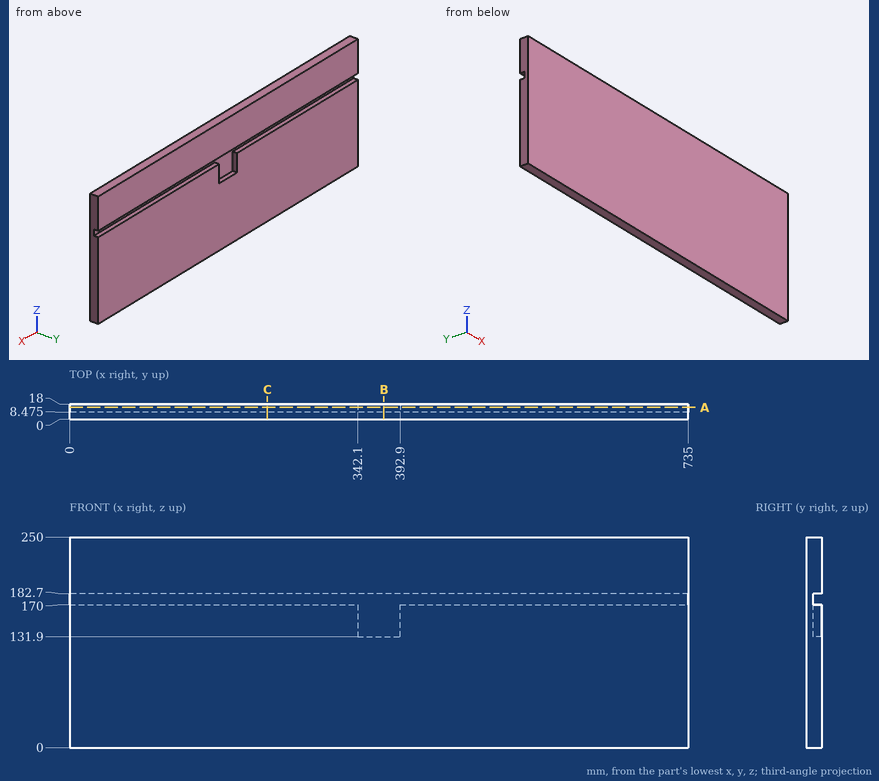
Job drawing, mm, ordinate dimensions from the low corner. One solid piece. Round coordinates to 2 decimals unless told otherwise and drop trailing zeros. Write each loop counter-clockwise with the first axis right and the second up, starting at its lowest first coordinate (ties: lowest second). Pieces come first, ordered by that corner, then holes.
1) Band-saw the part on B-B, the plane x = 373.5. List the corners of the cut face in (y, z) (3 decimals), and give its area (3 significant figures).
2) Band-saw the part on C-C, the plane x = 235. List the corners of the cut face in (y, z) (3 decimals).
3) Band-saw the part on A-A, the plane y = 14. List the corners of the cut face in (x, z).
4) Drill centre lines: probe 1 along Z at (x, y) = (194.5, 10.75); probe 2 along X at (y, z) = (8.75, 164); probe 3 along Z at (x, y) = (363.5, 13). Where is each one in solid material? Low to high.
Ans:
1. outline: (0, 0) - (18, 0) - (18, 131.9) - (8.475, 131.9) - (8.475, 182.7) - (18, 182.7) - (18, 250) - (0, 250) - close
1. area: 4,020 mm2
2. outline: (0, 0) - (18, 0) - (18, 170) - (8.475, 170) - (8.475, 182.7) - (18, 182.7) - (18, 250) - (0, 250) - close
3. outline: (0, 0) - (735, 0) - (735, 170) - (392.9, 170) - (392.9, 131.9) - (342.1, 131.9) - (342.1, 170) - (0, 170) - close; (0, 182.7) - (735, 182.7) - (735, 250) - (0, 250) - close
4. probe 1: z = 0 to 170, 182.7 to 250
4. probe 2: x = 0 to 342.1, 392.9 to 735
4. probe 3: z = 0 to 131.9, 182.7 to 250
